from build123d import *

# Parameters (mm, degrees)
F1_DEPTH = 25.4
F3_DEPTH = 25.4
F5_DEPTH = 25.4
F6_R     = 7.14088
F7_DEPTH = 25.4
F9_DEPTH = 25.4


with BuildPart() as f1:
    # F0 (on Front) → F1 (new body)
    with BuildSketch(Plane.XZ):
        Polygon((25.4, 38.1), (0, 38.1), (0, 0), (69.85, 0), (69.85, 12.7), (25.4, 12.7), align=None)
    extrude(amount=F1_DEPTH)

    # F2 (on face) → F3 (cut)
    with BuildSketch(Plane.XZ.offset(25.4)):
        with BuildLine():
            ThreePointArc((0, 31.003495), (12.683588, 37.919742), (25.4, 31.064033))
            Line((25.4, 31.064033), (25.4, 38.1))
            Line((25.4, 38.1), (0, 38.1))
            Line((0, 38.1), (0, 31.003495))
        make_face()
    extrude(amount=-F3_DEPTH, mode=Mode.SUBTRACT)

    # F4 (on face) → F5 (cut)
    with BuildSketch(Plane.XY.offset(12.7)):
        with BuildLine():
            ThreePointArc((63.532993, 0), (69.639018, -12.7), (63.532993, -25.4))
            Line((63.532993, -25.4), (69.85, -25.4))
            Line((69.85, -25.4), (69.85, 0))
            Line((69.85, 0), (63.532993, 0))
        make_face()
    extrude(amount=-F5_DEPTH, mode=Mode.SUBTRACT)

    # F6 (on face) → F7 (cut)
    with BuildSketch(Plane.XZ.offset(25.4)):
        with Locations((12.999689, 25.219742)):
            Circle(F6_R)
    extrude(amount=-F7_DEPTH, mode=Mode.SUBTRACT)

    # F8 (on face) → F9 (cut)
    with BuildSketch(Plane.XY.offset(12.7)):
        with BuildLine():
            Line((56.389028, -6.35), (38.564463, -6.35))
            ThreePointArc((38.564463, -6.35), (31.750977, -12.821492), (38.787275, -19.05))
            Line((38.787275, -19.05), (57.057447, -19.05))
            ThreePointArc((57.057447, -19.05), (63.280229, -12.354896), (56.389028, -6.35))
        make_face()
    extrude(amount=-F9_DEPTH, mode=Mode.SUBTRACT)


solid = f1.part
For this review, take the finished solid that the model builds, in its own axes (mm). A direction names the side the tool comes from. Round coordinates to 2 decimals unless told otherwise and drop trailing zeros. Write each loop counter-clockwise with the first axis right and the second up, starting at its lowest first coordinate (ties: lowest second). Pieces come first, ordered by that corner, then holes. Notation, with made-up numbers: (-3, -36.75) -> (33, -36.75) arc R18 ccw to (33, -10.75) -> close; hole circle Ø8 at (-37, 0). An arc over 180 degrees is marked (long way). Put each result on its own line as item: value.
Q1. Consider section D-D on z = 6. State the section outline as (x, y) points, and give its area (3 significant figures).
Determined:
outline: (0, -25.4) -> (63.53, -25.4) arc R16.26 ccw to (63.53, 0) -> (0, 0) -> close; hole (38.56, -6.35) arc R6.37 ccw (long way) to (38.79, -19.05) -> (57.06, -19.05) arc R6.36 ccw (long way) to (56.39, -6.35) -> close
area: 1,360 mm^2
Q2. To check wall thickness, follow L1, parallel to X at y = -13.5, z = 25; L2, parallel to X at y = -13.5, z = 12; L3, parallel to Z at x = 16, y = -16.75. State the ranges of each line that lie inside material, in increasing order. Write a range as [from, to].
Determined:
L1: x = [0, 5.86], [20.14, 25.4]
L2: x = [0, 31.8], [63.24, 69.62]
L3: z = [0, 18.74], [31.7, 37.56]
Q3. Consider section B-B on y = -10. State the section outline as (x, z) points.
Determined:
outline: (0, 0) -> (32.35, 0) -> (32.35, 12.7) -> (25.4, 12.7) -> (25.4, 31.06) arc R15.15 ccw to (0, 31) -> close; (62.69, 0) -> (69.41, 0) -> (69.41, 12.7) -> (62.69, 12.7) -> close; hole circle Ø14.28 at (13, 25.22)
Q4. Clearance check with flat-ended pins moving along their axes: pin 1 Ø1 at (y, z) = (-10, 7.5) entering from +X; pin 2 Ø4 at (y, z) = (-17.5, 17) entering from +X; pin 3 Ø1 at (x, y) = (49, -6.5) entering from +Z. State where each tip first meets the part, or that it passes through.
Determined:
pin 1: stops at x = 69.49
pin 2: stops at x = 25.4
pin 3: stops at z = 12.7
Q5. Consider section A-A on x = 51. State the section outline as (y, z) points, and give its area (3 significant figures).
Determined:
outline: (-25.4, 0) -> (-19.05, 0) -> (-19.05, 12.7) -> (-25.4, 12.7) -> close; (-6.35, 0) -> (0, 0) -> (0, 12.7) -> (-6.35, 12.7) -> close
area: 161 mm^2
Q6. Consider section C-C on z = 24. State the section outline as (x, y) points.
Determined:
outline: (0, -25.4) -> (5.96, -25.4) -> (5.96, 0) -> (0, 0) -> close; (20.04, -25.4) -> (25.4, -25.4) -> (25.4, 0) -> (20.04, 0) -> close
Q7. The part is to be moulded in two halves that separate along Y. For faces 4 (the flat face through (48, -19.05, 6)), 5 (the flat face through (27, -13, 0)), 6 (the flat face through (24, -25.4, 15)), 7 (the cylindrical face through (63.286, -12.498, 6.439)), say which applies: released by +Y, released by -Y, zero draft, split by the parting line, or undercut.
Determined:
face 4: undercut
face 5: zero draft
face 6: released by -Y
face 7: undercut
Q8. Machinability: for faces 1 (the cylindrical face through (31.75, -12.67, 6.44)), 2 (the cylindrical face through (12.473, -12.878, 37.918)), 3 (the flat face through (48, -4, 12.7)), which of the approach directions +Z, -Z, +X, -X, +Y, -Y give a long, thin tool a straight path to every point of the face, cutting with its end or side? Answer none if there is none.
Determined:
face 1: +Z, -Z
face 2: +Z, +Y, -Y
face 3: +Z, +X, +Y, -Y
